Autodesk Inventor part; units mm, degrees
ref_plane "YZ Plane" through (0, 0, 0) normal (1, 0, 0) x (0, 1, 0)
ref_plane "XZ Plane" through (0, 0, 0) normal (0, 1, 0) x (-1, 0, 0)
ref_plane "XY Plane" through (0, 0, 0) normal (0, 0, 1) x (1, 0, 0)
sketch "Esquisse12" plane through (0, 0, 0) normal (0, 0, 1) x (1, 0, 0)
  line L0 (0, 0) -> (20, 0)
  line L1 (20, 0) -> (20, 34)
  line L2 (20, 34) -> (0, 34)
  line L3 (0, 34) -> (0, 0)
  line L4 (10, 34) -> (10, 0) construction
  circle A0 centre (10, 5) radius 2.15
  line L5 (10, 5) -> (20, 5) construction
  circle A1 centre (16, 5) radius 2.15
  circle A2 centre (4, 5) radius 2.15
  circle A3 centre (10, 5) radius 2.15
  circle A4 centre (10, 23) radius 2.15
  circle A5 centre (16, 23) radius 2.15
  circle A6 centre (4, 23) radius 2.15
  dimension "d133" = 20
  dimension "d134" = 5
  dimension "d135" = 4.3
  dimension "d138" = 6
  dimension "d141" = 6
  dimension "d148" = 18
  dimension "d153" = 11
extrude "Extrusion13" add sketch "Esquisse12" along normal blind 2.2
fillet "Congé8" radius 7 2 edges at (20, 0, 1.1) (0, 0, 1.1)
mirror "Symétrie3" about plane through (20, 34, 0) normal (0, 1, 0)
equation "\"d135\" = Holes"
equation "\"d154\" = Depth"
equation "\"d156\" = Rounding"
equation "\"Depth\" = 2.2"
equation "\"Holes\" = 4.3"
equation "\"Height\" = 0"
equation "\"Rounding\" = 7"
properties part number "SideToSide"
Could you check a few things on this model? Use its own coordinates, in mm. Coordinates: 2 decimals unless noted, no trailing zeros. Write each loop counter-clockwise with the first axis right and the second up, starting at its lowest first coordinate (ties: lowest second). Pieces come first, ordered by that corner, then holes. Notation, with made-up numbers: (-4, 11) - (52, 11) arc R19 cw to (52, 42) - close; hole circle Ø10 at (61, 58.5). An arc over 180 degrees is marked (long way). Use a Markdown table: item, result.
Q1. Imagine slicing it at D-D (y = 63). List the corners of the cut face in (x, z) for me.
Geometry check:
| item | result |
|---|---|
| outline | (0.29, 0) - (1.85, 0) - (1.85, 2.2) - (0.29, 2.2) - close; (6.15, 0) - (7.85, 0) - (7.85, 2.2) - (6.15, 2.2) - close; (12.15, 0) - (13.85, 0) - (13.85, 2.2) - (12.15, 2.2) - close; (18.15, 0) - (19.71, 0) - (19.71, 2.2) - (18.15, 2.2) - close |
Q2. Imagine slicing it at B-B (z = 0.8). Count the separate pieces of the cut face and the enclosed holes in it, and give its area (3 significant figures).
Geometry check:
| item | result |
|---|---|
| separate pieces | 1 |
| enclosed holes | 12 |
| area | 1,140 mm2 |
Q3. I'm going to push flat-ended pins straight in: pin 1 Ø4 at (x, y) = (16, 45) entering from +Z; pin 2 Ø1 at (x, z) = (16.5, 1) entering from +Y. Where does each tip first touch, or does it pass through?
Geometry check:
| item | result |
|---|---|
| pin 1 | passes through |
| pin 2 | stops at y = 67.32 |
Q4. Thinking about a two-plate mould opening in X: for faces 1 (the flat face through (10, 34, 0)), 2 (the cylindrical face through (2, 2.1, 1.1)), 3 (the cylindrical face through (16.99, 24.91, 1.08)), 4 (the cylindrical face through (17.9, 2, 1.1)), which applies, +X half, -X half, draft (parallel to the pull), parting line (faces both ways), or undercut?
Geometry check:
| item | result |
|---|---|
| face 1 | draft |
| face 2 | -X half |
| face 3 | undercut |
| face 4 | +X half |
Q5. Imagine slicing it at C-C (y = 23). List the corners of the cut face in (x, z) for me.
Geometry check:
| item | result |
|---|---|
| outline | (0, 0) - (1.85, 0) - (1.85, 2.2) - (0, 2.2) - close; (6.15, 0) - (7.85, 0) - (7.85, 2.2) - (6.15, 2.2) - close; (12.15, 0) - (13.85, 0) - (13.85, 2.2) - (12.15, 2.2) - close; (18.15, 0) - (20, 0) - (20, 2.2) - (18.15, 2.2) - close |
Q6. Imagine slicing it at A-A (x = 10). List the corners of the cut face in (y, z) for me.
Geometry check:
| item | result |
|---|---|
| outline | (0, 0) - (2.85, 0) - (2.85, 2.2) - (0, 2.2) - close; (7.15, 0) - (20.85, 0) - (20.85, 2.2) - (7.15, 2.2) - close; (25.15, 0) - (42.85, 0) - (42.85, 2.2) - (25.15, 2.2) - close; (47.15, 0) - (60.85, 0) - (60.85, 2.2) - (47.15, 2.2) - close; (65.15, 0) - (68, 0) - (68, 2.2) - (65.15, 2.2) - close |
Q7. Please list where these lines run through material, in increasing order: L1, parallel to X at y = 45, z = 0.7; L2, parallel to Y at x = 14.75, z = 1.4; L3, parallel to X at y = 62.5, z = 0.45.
Geometry check:
| item | result |
|---|---|
| L1 | x = 0 to 1.85, 6.15 to 7.85, 12.15 to 13.85, 18.15 to 20 |
| L2 | y = 0.22 to 3.25, 6.75 to 21.25, 24.75 to 43.25, 46.75 to 61.25, 64.75 to 67.78 |
| L3 | x = 0.16 to 1.91, 6.09 to 7.91, 12.09 to 13.91, 18.09 to 19.84 |
